from build123d import *

# Parameters (mm, degrees)
SKETCH1_W           = 54.3999928
SKETCH1_H           = 27.5100034
BOSS_EXTRUDE1_DEPTH = 17.3500034
CUT_EXTRUDE1_DEPTH  = 15.3500074
CUT_EXTRUDE2_DEPTH  = 5.9200034
CUT_EXTRUDE3_DEPTH  = 9.430004
SKETCH5_W           = 4.795012
SKETCH5_H           = 2.9200094
CUT_EXTRUDE4_DEPTH  = 5.9200034
SKETCH6_W           = 2.769997
SKETCH6_H           = 3.499993
CUT_EXTRUDE5_DEPTH  = 15.3500074
CUT_EXTRUDE6_DEPTH  = 15.3500074
SKETCH8_R           = 1.7499965
CUT_EXTRUDE7_DEPTH  = 9.0000074
CUT_EXTRUDE8_DEPTH  = 13.9999974
SKETCH10_W          = 4.99999
SKETCH10_H          = 2.2999954
CUT_EXTRUDE9_DEPTH  = 4.320159
CUT_EXTRUDE10_DEPTH = 1.999996
CUT_EXTRUDE11_DEPTH = 2.999994
CUT_EXTRUDE12_DEPTH = 1.999996


with BuildPart() as part:
    # Sketch1 → Boss-Extrude1 (new body)
    with BuildSketch(Plane(origin=(0, 0, 0), x_dir=(1, 0, 0), z_dir=(0, 1, 0))):
        Rectangle(SKETCH1_W, SKETCH1_H)
    extrude(amount=BOSS_EXTRUDE1_DEPTH)

    # Sketch2 → Cut-Extrude1 (cut)
    with BuildSketch(Plane(origin=(0, 17.3500034, 0), x_dir=(1, 0, 0), z_dir=(0, 1, 0))):
        Polygon((-7.7499972, 12.7852805), (-20.7499966, 12.7852805), (-20.7499712, 8.7852885), (-21.699982, 8.7852885), (-21.699982, -1.2147169), (-25.9499862, -1.2147169), (-25.9499862, -12.5049915), (-24.199309728, -12.476075327), (-24.199309728, -7.476085327), (-22.999312128, -7.476085327), (-22.999312128, -3.2369379), (-16.999324128, -3.2369379), (-16.999324128, -7.2247379), (-15.799326528, -7.2247379), (-15.799326528, -11.2247299), (-7.569320128, -11.2247299), (-7.569320128, 3.8652831), (-12.364974, 3.8652831), (-12.364974, 9.2852875), (-7.5699874, 9.2852875), (-7.5699874, 10.5852849), (-7.7499972, 10.5852849), align=None)
    extrude(amount=-CUT_EXTRUDE1_DEPTH, mode=Mode.SUBTRACT)

    # Sketch3 → Cut-Extrude2 (cut)
    with BuildSketch(Plane(origin=(0, 17.3500034, 0), x_dir=(1, 0, 0), z_dir=(0, 1, 0))):
        Polygon((-7.5699874, -10.7550077), (-7.5699874, -1.7550003), (-6.3199772, -1.7550003), (-6.3199772, 11.7550057), (16.7300148, 11.7550057), (16.7300148, -10.7550077), align=None)
    extrude(amount=-CUT_EXTRUDE2_DEPTH, mode=Mode.SUBTRACT)

    # Sketch4 → Cut-Extrude3 (cut)
    with BuildSketch(Plane(origin=(0, 11.43, 0), x_dir=(1, 0, 0), z_dir=(0, 1, 0))):
        Polygon((15.2300178, 10.2550087), (15.2300178, -9.2549853), (-4.8199802, -9.2549853), (-4.8199802, 10.2550087), (-4.1839388, 10.2550087), (-4.1839388, 10.0550091), (-0.916671965, 10.0550091), (-0.916671965, 10.2550087), align=None)
    extrude(amount=-CUT_EXTRUDE3_DEPTH, mode=Mode.SUBTRACT)

    # Sketch5 → Cut-Extrude4 (cut)
    with BuildSketch(Plane(origin=(0, 17.3500034, 0), x_dir=(1, 0, 0), z_dir=(0, 1, 0))):
        with Locations((-8.7174832, 6.2949836)):
            Rectangle(SKETCH5_W, SKETCH5_H)
        with Locations((19.1275208, 6.2949836)):
            Rectangle(SKETCH5_W, SKETCH5_H)
    extrude(amount=-CUT_EXTRUDE4_DEPTH, mode=Mode.SUBTRACT)

    # Sketch6 → Cut-Extrude5 (cut)
    with BuildSketch(Plane(origin=(0, 17.3500034, 0), x_dir=(1, 0, 0), z_dir=(0, 1, 0))):
        with Locations((19.3649981, 10.754995)):
            Rectangle(SKETCH6_W, SKETCH6_H)
    extrude(amount=-CUT_EXTRUDE5_DEPTH, mode=Mode.SUBTRACT)

    # Sketch7 → Cut-Extrude6 (cut)
    with BuildSketch(Plane(origin=(0, 17.3500034, 0), x_dir=(1, 0, 0), z_dir=(0, 1, 0))):
        Polygon((21.7000074, 3.5849941), (17.9799996, 3.5849941), (17.9799996, -3.5050095), (23.0000048, -3.5050095), (23.0000048, -7.5050015), (24.2000024, -7.5050015), (24.2000024, -12.5049915), (25.9500116, -12.5049915), (25.9500116, -1.4949805), (21.7000074, -1.4949805), align=None)
    extrude(amount=-CUT_EXTRUDE6_DEPTH, mode=Mode.SUBTRACT)

    # Sketch8 → Cut-Extrude7 (cut)
    with BuildSketch(Plane.XY.offset(13.7550017)):
        with Locations((-19.9999981, 17.3500034)):
            Circle(SKETCH8_R)
        with Locations((19.9999981, 17.3500034)):
            Circle(SKETCH8_R)
    extrude(amount=-CUT_EXTRUDE7_DEPTH, mode=Mode.SUBTRACT)

    # Sketch9 → Cut-Extrude8 (cut)
    with BuildSketch(Plane(origin=(0, 0, -13.7550017), x_dir=(-1, 0, 0), z_dir=(0, 0, -1))):
        with BuildLine():
            Line((-25.4499872, 17.3500034), (-25.4499872, 14.2999968))
            ThreePointArc((-25.4499872, 14.2999968), (-24.1999897, 13.0499993), (-22.9499922, 14.2999968))
            Line((-22.9499922, 14.2999968), (-22.9499922, 17.3500034))
            Line((-22.9499922, 17.3500034), (-25.4499872, 17.3500034))
        make_face()
        with BuildLine():
            Line((22.9499922, 17.3500034), (25.4499872, 17.3500034))
            Line((25.4499872, 17.3500034), (25.4499872, 14.2999968))
            ThreePointArc((25.4499872, 14.2999968), (24.1999897, 13.0499993), (22.9499922, 14.2999968))
            Line((22.9499922, 14.2999968), (22.9499922, 17.3500034))
        make_face()
    extrude(amount=-CUT_EXTRUDE8_DEPTH, mode=Mode.SUBTRACT)

    # Sketch10 → Cut-Extrude9 (cut)
    with BuildSketch(Plane(origin=(0, 17.3500034, 0), x_dir=(1, 0, 0), z_dir=(0, 1, 0))):
        with Locations((-24.2000024, 10.754995)):
            Rectangle(SKETCH10_W, SKETCH10_H)
        with Locations((24.2000024, 10.754995)):
            Rectangle(SKETCH10_W, SKETCH10_H)
    extrude(amount=-CUT_EXTRUDE9_DEPTH, mode=Mode.SUBTRACT)

    # Sketch11 → Cut-Extrude10 (cut)
    with BuildSketch(Plane(origin=(0, 0, -11.7550057), x_dir=(-1, 0, 0), z_dir=(0, 0, -1))):
        Polygon((-26.399998, 13.0298444), (-24.2000024, 11.7596666), (-22.0000068, 13.0298444), align=None)
        Polygon((22.0000068, 13.0298444), (24.2000024, 11.7596666), (26.399998, 13.0298444), align=None)
    extrude(amount=-CUT_EXTRUDE10_DEPTH, mode=Mode.SUBTRACT)

    # Sketch13 → Cut-Extrude11 (cut)
    with BuildSketch(Plane.XY.offset(11.7550057)):
        Polygon((-22.9581964, 17.3500034), (-17.0581828, 17.3500034), (-17.0581828, 15.6468318), (-20.0081896, 13.9436602), (-22.9581964, 15.6468318), align=None)
        Polygon((17.0581828, 15.6468318), (20.0081896, 13.9436602), (22.9581964, 15.6468318), (22.9581964, 17.3500034), (17.0581828, 17.3500034), align=None)
    extrude(amount=-CUT_EXTRUDE11_DEPTH, mode=Mode.SUBTRACT)

    # Sketch14 → Cut-Extrude12 (cut)
    with BuildSketch(Plane(origin=(0, 0, -13.7550017), x_dir=(-1, 0, 0), z_dir=(0, 0, -1))):
        with BuildLine():
            Line((-6.499990556, 17.3500034), (-8.8399874, 17.3500034))
            ThreePointArc((-8.8399874, 17.3500034), (-7.917895682, 15.129395373), (-5.694061964, 14.215110549))
            ThreePointArc((-5.694061964, 14.215110549), (-6.295284996, 15.731587965), (-6.499990556, 17.3500034))
        make_face()
        with BuildLine():
            Line((-2.570163008, 17.3500034), (-6.499990556, 17.3500034))
            ThreePointArc((-6.499990556, 17.3500034), (-6.295284996, 15.731587965), (-5.694061964, 14.215110549))
            ThreePointArc((-5.694061964, 14.215110549), (-3.484467177, 15.137182922), (-2.570163008, 17.3500034))
        make_face()
        with BuildLine():
            ThreePointArc((-2.570163008, 17.3500034), (-3.484467177, 15.137182922), (-5.694061964, 14.215110549))
            ThreePointArc((-5.694061964, 14.215110549), (1.618426357, 11.054707482), (6.5000124, 17.3500034))
            Line((6.5000124, 17.3500034), (-2.570163008, 17.3500034))
        make_face()
    extrude(amount=-CUT_EXTRUDE12_DEPTH, mode=Mode.SUBTRACT)


solid = part.part
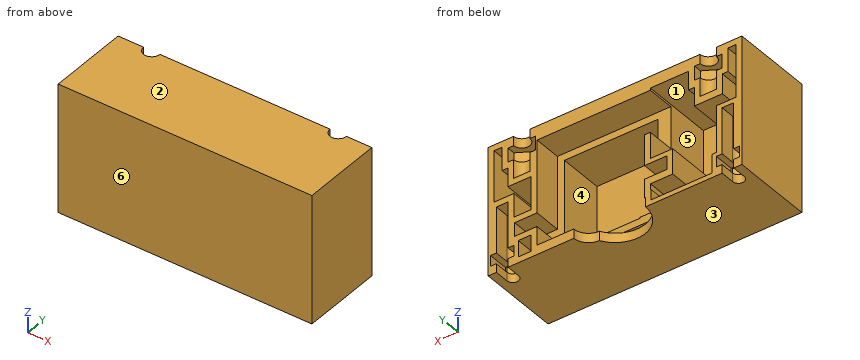
Geometry: final body of the model. Coordinates: model frame, mm. Face numbers are marked on the shaded views. A direction names the side the tool comes from. Coordinates: 2 decimals unless noted, no trailing zeros. Order: outer loops, then holes, each group sorted by start corner. A loop starts at its lowest first (then second) coordinate and runs counter-clockwise, first axis right, second up.
(1) Section query D-D (z = -2.25). Return the cut outline in (x, y), plus the area to 3 significant figures.
(2) Section query A-A (z = 2.5). Return the cut outline in (x, y), plus the area to 3 significant figures.
(3) Section query C-C (y = 4.75). State how many separate pieces and enclosed holes the cut face has, plus the area to 3 significant figures.
(4) Section query B-B (x = 10). Return the cut outline in (y, z) (3 decimals).
(5) Draft query along Z for the marked faces 3, 4, 5 and 6. Return one class per face: pulls with the +Z half, pulls with the -Z half, needs draft (parallel to the pull), parting line crosses it, or undercut.
(6) First-contact query: pin 1 (10 mm diameter, centred on x = 4, z = 1, fed in from +Y). Flat tip, straight axial feed; report the tip coordinate or a pass-through.
(7) Access query for the marked faces 1 and 2. Directions: +Z, -Z, +X, -X, +Y, -Y. A direction counts if a zero-diameter tool reaches every point of the face in a straight line with its end or side. Return the directions, or none.
(8) Material intervals for probe 1 along Z at (x, y) = (19.5, 5.25) (3 decimals); probe 2 along X at (y, z) = (7.25, -6.5); probe 3 along X at (y, z) = (13.5, 8.25), sorted ascending.
Solution:
1. outline: (-27.2, 0) - (27.2, 0) - (27.2, 17.35) - (25.45, 17.35) - (25.45, 14.3) arc R1.25 cw to (22.95, 14.3) - (22.95, 17.35) - (21.7, 17.35) - (21.7, 2) - (17.98, 2) - (17.98, 17.35) - (16.73, 17.35) - (16.73, 11.43) - (15.23, 11.43) - (15.23, 2) - (-4.82, 2) - (-4.82, 11.43) - (-6.32, 11.43) - (-6.32, 17.35) - (-7.57, 17.35) - (-7.57, 2) - (-21.7, 2) - (-21.7, 17.35) - (-22.95, 17.35) - (-22.95, 14.3) arc R1.25 cw to (-25.45, 14.3) - (-25.45, 17.35) - (-27.2, 17.35) - close
1. area: 324 mm2
2. outline: (-27.2, 0) - (27.2, 0) - (27.2, 17.35) - (25.95, 17.35) - (25.95, 2) - (17.98, 2) - (17.98, 17.35) - (16.73, 17.35) - (16.73, 11.43) - (15.23, 11.43) - (15.23, 2) - (-4.82, 2) - (-4.82, 11.43) - (-7.57, 11.43) - (-7.57, 2) - (-25.95, 2) - (-25.95, 17.35) - (-27.2, 17.35) - close
2. area: 206 mm2
3. separate pieces: 1
3. enclosed holes: 4
3. area: 744 mm2
4. outline: (0, -13.755) - (17.35, -13.755) - (17.35, -11.755) - (11.43, -11.755) - (11.43, -10.255) - (2, -10.255) - (2, 9.255) - (11.43, 9.255) - (11.43, 10.755) - (17.35, 10.755) - (17.35, 13.755) - (0, 13.755) - close
5. face 3: pulls with the -Z half
5. face 4: undercut
5. face 5: undercut
5. face 6: needs draft
6. pin 1: stops at y = 2
7. face 1: +Y
7. face 2: +Z, +X, -X, +Y, -Y
8. probe 1: z = -13.755 to -12.505, -9.005 to -3.585, 3.505 to 13.755
8. probe 2: x = -27.2 to -21.7, -12.36 to -4.82, 15.23 to 27.2
8. probe 3: x = -27.2 to -25.95, -24.2 to -15.8, 16.73 to 24.2, 25.95 to 27.2
